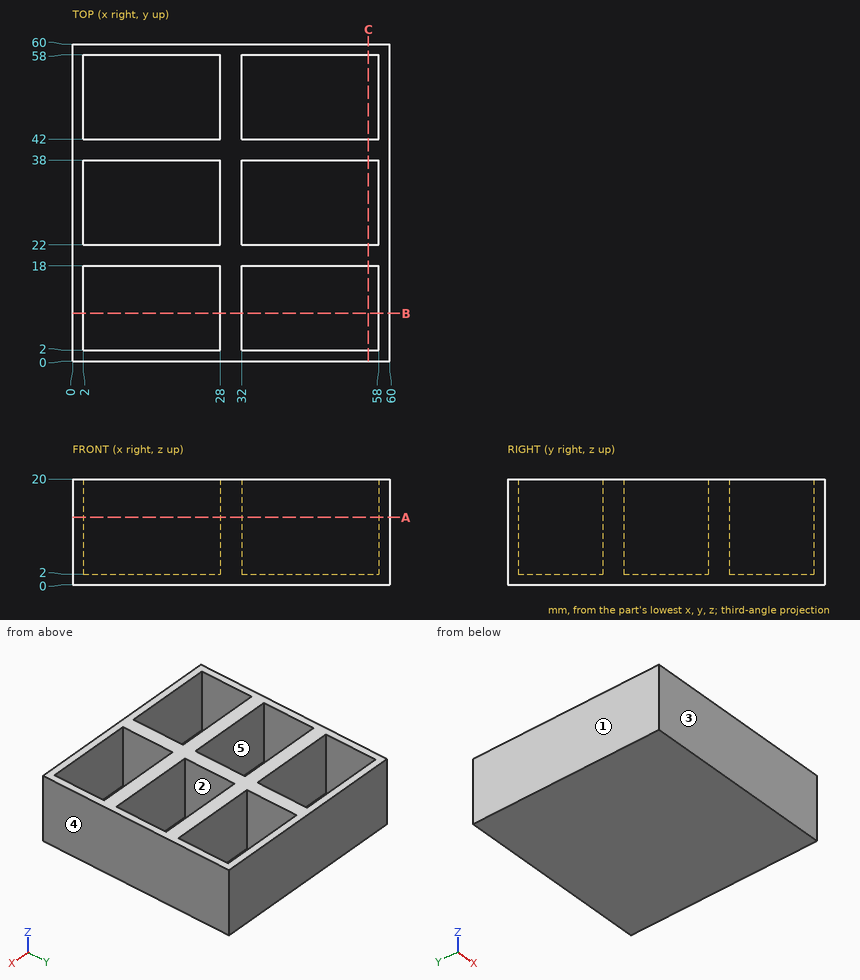
Geometry check sheet. Reference: drawing and pictorial views, mm from the part's lowest x, y, z. A direction names the side the tool comes from. Give positions to 0.01 mm unless a question says otherwise; leave off trailing zeros. Order: outer loops, then holes, each group sorted by start corner. A loop starts at its lowest first (then second) coordinate and runs counter-clockwise, first axis right, second up. Notation, with made-up numbers: M 69,43 L 106,43 A21 cw 106,80 Z; hole C -28,81.5 d10. An arc over 180 degrees is marked long. Answer in a Markdown table with one row per item. Add a question column.
Q1. Gauge pin test, flat ends, axial feed: pin 1 Ø3 at (y, z) = (43, 13) entering from -X; pin 2 Ø5 at (x, y) = (13, 47) entering from +Z. Record the tip position at first contact, or that the pin passes through.
Q2. Release check for a two-part mould opening along X. For the marked faces 3, 4 and 5 record: released by +X, released by -X, zero draft, split by the parting line, or undercut.
Q3. Access from +Z, -Z, +X, -X, +Y, -Y to the whole of each face (thin tool, end or side, straight path). Record for the marked faces 1 and 2.
Q4. Sectioned sample at A-A, the plane z = 12.75. Record the boundary of the cut face in (x, y).
Q5. Thickness scan on L1, parallel to X at y = 7.5, z = 4.75; L2, parallel to Y at x = 56.5, z = 19; L3, parallel to Z at x = 13, y = 13.5. Record the ranges inside material, lowest first.
Q6. Sectioned sample at C-C, the plane x = 56. Record the boundary of the cut face in (y, z).
Q7. Sectioned sample at B-B, the plane y = 9. Record the boundary of the cut face in (x, z).
Verdict:
| question | item | result |
|---|---|---|
| 1 | pin 1 | x = 0 |
| 1 | pin 2 | z = 2 |
| 2 | face 3 | zero draft |
| 2 | face 4 | released by +X |
| 2 | face 5 | undercut |
| 3 | face 1 | +Z, -Z, -X, +Y, -Y |
| 3 | face 2 | +Z |
| 4 | outline | M 0,0 L 60,0 L 60,60 L 0,60 Z; hole M 2,2 L 28,2 L 28,18 L 2,18 Z; hole M 2,22 L 28,22 L 28,38 L 2,38 Z; hole M 2,42 L 28,42 L 28,58 L 2,58 Z; hole M 32,2 L 58,2 L 58,18 L 32,18 Z; hole M 32,22 L 58,22 L 58,38 L 32,38 Z; hole M 32,42 L 58,42 L 58,58 L 32,58 Z |
| 5 | L1 | 0 to 2, 28 to 32, 58 to 60 |
| 5 | L2 | 0 to 2, 18 to 22, 38 to 42, 58 to 60 |
| 5 | L3 | 0 to 2 |
| 6 | outline | M 0,0 L 60,0 L 60,20 L 58,20 L 58,2 L 42,2 L 42,20 L 38,20 L 38,2 L 22,2 L 22,20 L 18,20 L 18,2 L 2,2 L 2,20 L 0,20 Z |
| 7 | outline | M 0,0 L 60,0 L 60,20 L 58,20 L 58,2 L 32,2 L 32,20 L 28,20 L 28,2 L 2,2 L 2,20 L 0,20 Z |
